```python
from build123d import *

# Parameters (mm, degrees)
BOSS_EXTRUDE1_DEPTH = 60
FILLET1_R           = 15
FILLET2_R           = 8
SKETCH2_R           = 12.5
CUT_EXTRUDE1_DEPTH  = 100
SKETCH4_W           = 25.4
SKETCH4_H           = 25.4
CUT_EXTRUDE2_DEPTH  = 0.1


with BuildPart() as part:
    # Sketch1 → Boss-Extrude1 (new body)
    with BuildSketch(Plane.XY):
        Polygon((0, -37.5), (0, 37.5), (60, 37.5), (60, 27.5), (10, 27.5), (10, -27.5), (60, -27.5), (60, -37.5), align=None)
    extrude(amount=BOSS_EXTRUDE1_DEPTH)

    # Fillet1
    fillet1_edges = [part.edges().sort_by_distance(p)[0] for p in [
        (60, -32.5, 0),
        (60, -32.5, 60),
        (60, 32.5, 60),
        (60, 32.5, 0),
    ]]
    fillet(fillet1_edges, radius=FILLET1_R)

    # Fillet2
    fillet2_edges = [part.edges().sort_by_distance(p)[0] for p in [
        (10, 27.5, 30),
        (10, -27.5, 30),
        (0, -37.5, 30),
        (0, 37.5, 30),
    ]]
    fillet(fillet2_edges, radius=FILLET2_R)

    # Sketch2 → Cut-Extrude1 (cut)
    with BuildSketch(Plane(origin=(0, 37.5, 0), x_dir=(1, 0, 0), z_dir=(0, 1, 0))):
        with Locations(Location((33, -30, 0), (0, 0, 270))):
            Circle(SKETCH2_R)
    extrude(amount=-CUT_EXTRUDE1_DEPTH, mode=Mode.SUBTRACT)

    # Sketch4 → Cut-Extrude2 (cut)
    with BuildSketch(Plane.ZY):
        with Locations((30, 0)):
            Rectangle(SKETCH4_W, SKETCH4_H)
    extrude(amount=-CUT_EXTRUDE2_DEPTH, mode=Mode.SUBTRACT)


solid = part.part
```
Work out the finished part from the listing and answer in its coordinate system (mm). A direction names the side the tool comes from. Give positions to 0.01 mm unless a question says otherwise; leave off trailing zeros. Write each loop counter-clockwise with the first axis right and the second up, starting at its lowest first coordinate (ties: lowest second). Pieces come first, ordered by that corner, then holes. Notation, with made-up numbers: (27, 51) -> (51, 51) arc R22 ccw to (51, 61) -> close; hole circle Ø7 at (-14.75, 27). An arc over 180 degrees is marked (long way). Write each question's results on one line, items separated by ' | '.
1. Find section A-A on z = 30. Determine the outline of the cut face in (x, y), and give its area (3 significant figures).
Data:
outline: (0, -29.5) arc R8 ccw to (8, -37.5) -> (20.5, -37.5) -> (20.5, -27.5) -> (18, -27.5) arc R8 cw to (10, -19.5) -> (10, 19.5) arc R8 cw to (18, 27.5) -> (20.5, 27.5) -> (20.5, 37.5) -> (8, 37.5) arc R8 ccw to (0, 29.5) -> (0, 12.7) -> (0.1, 12.7) -> (0.1, -12.7) -> (0, -12.7) -> close; (45.5, -37.5) -> (60, -37.5) -> (60, -27.5) -> (45.5, -27.5) -> close; (45.5, 27.5) -> (60, 27.5) -> (60, 37.5) -> (45.5, 37.5) -> close | area: 1,250 mm^2
2. Each of these flat-tipped pins is pushed along its axis until it touches: pin 1 Ø12.5 at (x, z) = (37.5, 28) entering from -Y; pin 2 Ø6 at (y, z) = (22.5, 7.5) entering from +X; pin 3 Ø5 at (y, z) = (9, 51) entering from +X. Where does it stop, or does it pass through?
Data:
pin 1: through | pin 2: x = 12.71 | pin 3: x = 10
3. Determine the mould class of faces 4 (the cylindrical face through (2.281, -35.094, 30.42)), 5 (the cylindrical face through (12.281, -25.094, 30.42)), 6 (the cylindrical face through (25.394, -32.43, 20.08)) for opening direction X: +X half, -X half, draft (parallel to the pull), parting line (faces both ways), or undercut.
Data:
face 4: -X half | face 5: +X half | face 6: undercut
4. Find section D-D on y = 5. Determine the outline of the cut face in (x, z).
Data:
outline: (0, 0) -> (10, 0) -> (10, 60) -> (0, 60) -> (0, 42.7) -> (0.1, 42.7) -> (0.1, 17.3) -> (0, 17.3) -> close
5. Find section B-B on x = 33. Determine the outline of the cut face in (y, z).
Data:
outline: (-37.5, 0) -> (-27.5, 0) -> (-27.5, 17.5) -> (-37.5, 17.5) -> close; (-37.5, 42.5) -> (-27.5, 42.5) -> (-27.5, 60) -> (-37.5, 60) -> close; (27.5, 0) -> (37.5, 0) -> (37.5, 17.5) -> (27.5, 17.5) -> close; (27.5, 42.5) -> (37.5, 42.5) -> (37.5, 60) -> (27.5, 60) -> close
6. Straight lines are drawn through the part: L1, parallel to Y at x = 44, z = 37; L2, parallel to X at y = -13, z = 41; L3, parallel to X at y = 35.75, z = 30. For each, find the intervals that lie inside material, in ascending order.
Data:
L1: -37.5 to -27.5, 27.5 to 37.5 | L2: 0 to 10 | L3: 3.01 to 20.5, 45.5 to 60
7. Find section C-C on x = 47. Determine the outline of the cut face in (y, z), and give its area (3 significant figures).
Data:
outline: (-37.5, 0.13) -> (-27.5, 0.13) -> (-27.5, 59.87) -> (-37.5, 59.87) -> close; (27.5, 0.13) -> (37.5, 0.13) -> (37.5, 59.87) -> (27.5, 59.87) -> close | area: 1,190 mm^2
8. A tool of negligible diameter and unlimited length cuts with its end or side. For faces 1 (the cylindrical face through (55.72, -32.57, 4.51)), 2 (the flat face through (10, 0, 30)), 3 (the flat face through (0.1, 0, 30)), from which of +Z, -Z, +X, -X, +Y, -Y can it reach the whole face along a straight path? Write none if from no direction.
Data:
face 1: -Z, +X, +Y, -Y | face 2: +Z, -Z, +X | face 3: -X
